```python
from build123d import *

# Parameters (mm, degrees)
F0_W           = 95
F0_H           = 35
F1_DEPTH       = 3.5
F2_SIZE        = 5
F4_DEPTH       = 2
F5_R           = 5.25
F7_DEPTH       = 2
F8_D           = 3.3
F8_CSINK_D     = 8
F8_CSINK_ANGLE = 90
F9_SIZE        = 1.5


with BuildPart() as f1:
    # F0 (on Front) → F1 (new body)
    with BuildSketch(Plane.XZ):
        Rectangle(F0_W, F0_H)
    extrude(amount=F1_DEPTH)

    # F2
    f2_edges = [f1.edges().sort_by_distance(p)[0] for p in [
        (47.5, -1.75, -17.5),
        (47.5, -1.75, 17.5),
        (-47.5, -1.75, -17.5),
        (-47.5, -1.75, 17.5),
    ]]
    chamfer(f2_edges, length=F2_SIZE)

    # F3 (on face) → F4 (cut)
    with BuildSketch(Plane.XZ.offset(3.5)):
        Polygon((41.6715728753, 15.5), (-41.6715728753, 15.5), (-45.5, 11.6715728753), (-45.5, -11.6715728753), (-41.6715728753, -15.5), (41.6715728753, -15.5), (45.5, -11.6715728753), (45.5, 11.6715728753), align=None)
    extrude(amount=-F4_DEPTH, mode=Mode.SUBTRACT)

    # F5 (on face) → F7 (join, through all)
    with BuildSketch(Plane.XZ.offset(3.5)):
        with Locations((33, 0)):
            Circle(F5_R)
        with Locations((-33, 0)):
            Circle(F5_R)
    extrude(amount=-F7_DEPTH)

    # F8 (through all)
    with Locations(Plane(origin=(0, 0, 0), x_dir=(-1, 0, 0), z_dir=(0, 1, 0))):
        with Locations((33, 0), (-32.9310148954, 0)):
            CounterSinkHole(F8_D / 2, F8_CSINK_D / 2, counter_sink_angle=F8_CSINK_ANGLE)

    # F9
    f9_edges = [f1.edges().sort_by_distance(p)[0] for p in [
        (0, 0, -17.5),
        (45, 0, -15),
        (47.5, 0, 0),
        (45, 0, 15),
        (0, 0, 17.5),
        (-45, 0, 15),
        (-45, 0, -15),
        (-47.5, 0, 0),
    ]]
    chamfer(f9_edges, length=F9_SIZE)


solid = f1.part
```
Could you check a few things on this model? Use its own coordinates, in mm. A direction names the side the tool comes from. Round coordinates to 2 decimals unless told otherwise and drop trailing zeros. Loops run counter-clockwise (first coordinate to the right, second up) from the corner with the lowest first, then second, coordinate; pieces in that order, holes last. Notation, with made-up numbers: (78, -2) - (129, -2) arc R21 cw to (129, 11) - close; hole circle Ø1 at (84.5, 33). An arc over 180 degrees is marked (long way). Use CSV: the item, a comma, the result in double quotes.
Item 1: If we section it at A-A on x = -33: List the corners of the cut face in (y, z) for me, then the cut area to 3 significant figures.
Here are the results:
outline,"(-3.5, -17.5) - (-1.5, -17.5) - (0, -16) - (0, -4) - (-2.35, -1.65) - (-3.5, -1.65) - (-3.5, -5.25) - (-1.5, -5.25) - (-1.5, -15.5) - (-3.5, -15.5) - close; (-3.5, 1.65) - (-2.35, 1.65) - (0, 4) - (0, 16) - (-1.5, 17.5) - (-3.5, 17.5) - (-3.5, 15.5) - (-1.5, 15.5) - (-1.5, 5.25) - (-3.5, 5.25) - close"
area,"62.2 mm²"
Item 2: Will these pins go through, and if not, where does the flat tip stop? pin 1 (1 mm diameter, centred on x = 29, y = -0.5, fed in from +Z); pin 2 (4 mm diameter, centred on x = 28.5, z = 6.5, fed in from -Y).
Here are the results:
pin 1,"stops at z = 17"
pin 2,"stops at y = -1.5"
Item 3: I need wall thicknesses on L1, parallel to Z at x = -33, y = -3.15; L2, parallel to Z at x = 4, y = -2.9; L3, parallel to X at y = -2.7, z = -8. Which ranges of each line are inside material? Lowest first, please. Write a range as [from, to].
Here are the results:
L1,"z = [-17.5, -15.5], [-5.25, -1.65], [1.65, 5.25], [15.5, 17.5]"
L2,"z = [-17.5, -15.5], [15.5, 17.5]"
L3,"x = [-47.5, -45.5], [45.5, 47.5]"
Item 4: If we mould it in two halves opening along X, with no side actions, what happens to faces 1 (the flat face through (-45, -2, 15)), 2 (the flat face through (-1, 0, 0)), 3 (the conical face through (34.61, -2.24, 0.53))? For each: pulls with the +X half, pulls with the -X half, needs draft (parallel to the pull), parting line crosses it, or undercut.
Here are the results:
face 1,"pulls with the -X half"
face 2,"needs draft"
face 3,"undercut"
Item 5: For faces 4 (the cylindrical face through (27.755, -2.514, 0.231)), 5 (the cylindrical face through (31.283, -2.933, 0.073)), which set-ups out of +Z, -Z, +X, -X, +Y, -Y let a thin tool reach every point of the face, with its end or its side?
Here are the results:
face 4,"-Y"
face 5,"+Y, -Y"
Item 6: If we section it at D-D on y = -0.7: List the corners of the cut face in (x, z) for me, then the cut area to 3 significant figures.
Here are the results:
outline,"(-46.7, -12.17) - (-42.17, -16.7) - (42.17, -16.7) - (46.7, -12.17) - (46.7, 12.17) - (42.17, 16.7) - (-42.17, 16.7) - (-46.7, 12.17) - close; hole circle Ø6.6 at (-33, 0); hole circle Ø6.6 at (32.93, 0)"
area,"3,010 mm²"
Item 7: If we section it at C-C on x = 11.5: List the corners of the cut face in (y, z) for me.
Here are the results:
outline,"(-3.5, -17.5) - (-1.5, -17.5) - (0, -16) - (0, 16) - (-1.5, 17.5) - (-3.5, 17.5) - (-3.5, 15.5) - (-1.5, 15.5) - (-1.5, -15.5) - (-3.5, -15.5) - close"
Item 8: If we section it at B-B on z = 0: Count the separate pieces of the cut face and the enclosed holes in it, then the cut area to 3 significant figures.
Here are the results:
separate pieces,"3"
enclosed holes,"0"
area,"156 mm²"
